Verification items for the finished model (mm, model axes). Face numbers are marked on the shaded views. A direction names the side the tool comes from. Give positions to 0.01 mm unless a question says otherwise; leave off trailing zeros. Write each loop counter-clockwise with the first axis right and the second up, starting at its lowest first coordinate (ties: lowest second). Pieces come first, ordered by that corner, then holes. Notation, with made-up numbers: (-11.5, 8) -> (11.5, 8) arc R9 ccw to (11.5, 21) -> close; hole circle Ø4 at (0.5, 24). An arc over 180 degrees is marked (long way). Answer as CSV lines item,"result". Start each with the question number.
1) Tool access check on the marked faces 1 and 2. Record the directions out of +Z, -Z, +X, -X, +Y, -Y that give a thin tool (end or side, any length) a straight path to the whole face; none if there is none.
2) Sectioned sample at A-A on z = 8. Record the cut outline in (x, y).
3) Sectioned sample at B-B on y = 25.5. Record the cut outline in (x, z), and give its area (3 significant figures).
4) Sectioned sample at D-D on y = 6. Give the number of separate pieces and of enclosed holes in the cut face, and give its area (3 significant figures).
5) Sectioned sample at C-C on y = 41.5. Record the cut outline in (x, z).
6) Gauge pin test, flat ends, axial feed: pin 1 Ø12 at (y, z) = (38.5, 6) entering from +X; pin 2 Ø0.9 at (x, z) = (46.5, 13.5) entering from +Y; pin 3 Ø3 at (x, y) = (18.5, 67.5) entering from +Z. Record the tip position at first contact, or that the pin passes through.
7) Material ranges on L1, parallel to X at y = 43.5, z = 4.75; L2, parallel to Z at x = 31, y = 8; L3, parallel to Y at x = 52.5, z = 10.75, recorded low to high.
```python
from build123d import *

# Parameters (mm, degrees)
BOSS_EXTRUDE1_DEPTH             = 10
SKIZZE2_W                       = 75
SKIZZE2_H                       = 9
AUFSATZ_LINEAR_AUSTRAGEN1_DEPTH = 10
SCHNITT_LINEAR_AUSTRAGEN2_DEPTH = 10
AUFSATZ_LINEAR_AUSTRAGEN2_DEPTH = 3


with BuildPart() as part:
    # Sketch1 → Boss-Extrude1 (new body)
    with BuildSketch(Plane.XY):
        with BuildLine():
            Line((7, 0), (0, 0))
            Line((0, 0), (0, 47.7))
            Line((0, 47.7), (0, 55))
            ThreePointArc((0, 55), (8.786796564, 76.213203436), (30, 85))
            Line((30, 85), (32, 85))
            Line((32, 85), (32, 65))
            Line((32, 65), (22, 65))
            ThreePointArc((22, 65), (11.393398282, 60.606601718), (7, 50))
            Line((7, 50), (7, 0))
        make_face()
    extrude(amount=BOSS_EXTRUDE1_DEPTH)

    # Skizze2 → Aufsatz-Linear austragen1 (add)
    with BuildSketch(Plane.XY.offset(10)):
        with Locations((37.5, 4.5)):
            Rectangle(SKIZZE2_W, SKIZZE2_H)
    extrude(amount=AUFSATZ_LINEAR_AUSTRAGEN1_DEPTH)

    # Skizze3 → Schnitt-Linear austragen2 (cut)
    with BuildSketch(Plane.XY.offset(20)):
        Polygon((3.370852377, 4.4746), (1.647110898, 4.4746), (0, 9), (5.017963275, 9), align=None)
        Polygon((9.670852377, 4.4746), (7.947110898, 4.4746), (6.3, 9), (11.317963275, 9), align=None)
        Polygon((15.970852377, 4.4746), (14.247110898, 4.4746), (12.6, 9), (17.617963275, 9), align=None)
        Polygon((22.270852377, 4.4746), (20.547110898, 4.4746), (18.9, 9), (23.917963275, 9), align=None)
        Polygon((28.570852377, 4.4746), (26.847110898, 4.4746), (25.2, 9), (30.217963275, 9), align=None)
        Polygon((34.870852377, 4.4746), (33.147110898, 4.4746), (31.5, 9), (36.517963275, 9), align=None)
        Polygon((41.170852377, 4.4746), (39.447110898, 4.4746), (37.8, 9), (42.817963275, 9), align=None)
        Polygon((47.470852377, 4.4746), (45.747110898, 4.4746), (44.1, 9), (49.117963275, 9), align=None)
        Polygon((53.770852377, 4.4746), (52.047110898, 4.4746), (50.4, 9), (55.417963275, 9), align=None)
        Polygon((60.070852377, 4.4746), (58.347110898, 4.4746), (56.7, 9), (61.717963275, 9), align=None)
        Polygon((66.370852377, 4.4746), (64.647110898, 4.4746), (63, 9), (68.017963275, 9), align=None)
        Polygon((72.670852377, 4.4746), (70.947110898, 4.4746), (69.3, 9), (74.317963275, 9), align=None)
    extrude(amount=-SCHNITT_LINEAR_AUSTRAGEN2_DEPTH, mode=Mode.SUBTRACT)

    # Skizze4 → Aufsatz-Linear austragen2 (add)
    with BuildSketch(Plane.ZY):
        Polygon((20, 0), (0, 0), (0, 48), (10, 48), (10, 38), (20, 38), align=None)
    extrude(amount=-AUFSATZ_LINEAR_AUSTRAGEN2_DEPTH)


solid = part.part
```
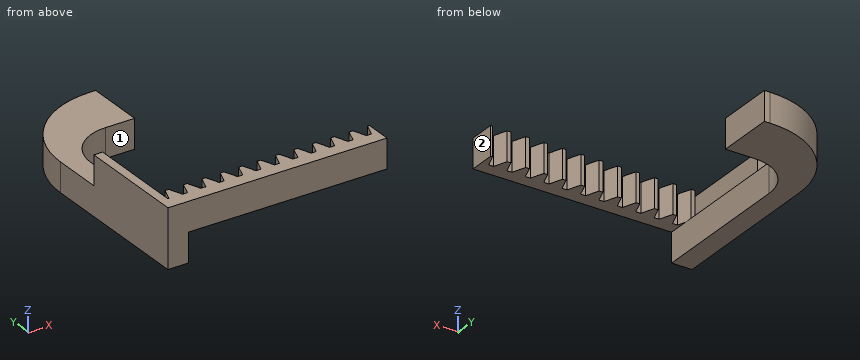
Ans:
1,face 1,"+Z, -Z, +X, -Y"
1,face 2,"+Z, -Z, +X, +Y, -Y"
2,outline,"(0, 0) -> (7, 0) -> (7, 50) arc R15 cw to (22, 65) -> (32, 65) -> (32, 85) -> (30, 85) arc R30 ccw to (0, 55) -> close"
3,outline,"(0, 0) -> (7, 0) -> (7, 10) -> (3, 10) -> (3, 20) -> (0, 20) -> close"
3,area,"100 mm²"
4,separate pieces,"12"
4,enclosed holes,"0"
4,area,"499 mm²"
5,outline,"(0, 0) -> (7, 0) -> (7, 10) -> (0, 10) -> close"
6,pin 1,"stops at x = 7"
6,pin 2,"stops at y = 4.47"
6,pin 3,"stops at z = 10"
7,L1,"x = 0 to 7"
7,L2,"z = 10 to 20"
7,L3,"y = 0 to 4.47"
